Design review of the part built by this model. Coordinates are the model's own, in mm. A direction names the side the tool comes from. Give positions to 0.01 mm unless a question says otherwise; leave off trailing zeros. Loops run counter-clockwise (first coordinate to the right, second up) from the corner with the lowest first, then second, coordinate; pieces in that order, holes last. Notation, with made-up numbers: (81, -25) - (137, -25) arc R38 ccw to (137, 13) - close; hole circle Ø7 at (-6, 89). An arc over 180 degrees is marked (long way). Write each question's results on one line, items separated by ' | '.
Autodesk Inventor part; units mm, degrees
ref_plane "Work Plane1" through (0, 0, 9) normal (0, 0, 1) x (1, 0, 0)
ref_plane "Work Plane2" through (-9, 0, 0) normal (1, 0, 0) x (0, 1, 0)
ref_plane "XZ Plane" through (0, 0, 0) normal (0, 1, 0) x (-1, 0, 0)
sketch "Sketch1" plane through (0, 0, 0) normal (0, 1, 0) x (-1, 0, 0)
  circle A0 centre (0, 0) radius 12.5
  dimension "d0" = 25
extrude "Extrusion1" add sketch "Sketch1" along normal blind 1
chamfer "Chamfer1" distance 0.4 angle 45 1 edges at (12.5, 1, 0)
sketch "Sketch2" plane through (0, 1, 0) normal (0, 1, 0) x (1, 0, 0)
  circle A0 centre (0, 0) radius 12.1
  circle A1 centre (0, 0) radius 9.9
  dimension "d6" = 19.8
extrude "Extrusion2" add sketch "Sketch2" along normal blind 6.5 contours A1
sketch "Sketch3" plane through (0, 7.5, 0) normal (0, 1, 0) x (1, 0, 0)
  circle A0 centre (0, 0) radius 12.5
extrude "Extrusion3" add sketch "Sketch3" along normal blind 1
sketch "Sketch4" plane through (0, 8.5, 0) normal (0, 1, 0) x (1, 0, 0)
  circle A0 centre (0, 0) radius 8.75
  dimension "d14" = 17.5
extrude "Extrusion4" add sketch "Sketch4" along normal blind 9
sketch "Sketch5" plane through (0, 17.5, 0) normal (0, 1, 0) x (1, 0, 0)
  circle A0 centre (0, 0) radius 8.75
  circle A1 centre (0, 0) radius 2.5
  dimension "d17" = 5
extrude "Extrusion5" cut sketch "Sketch5" against normal up to surface (17.5 mm away) contours A1
sketch "Sketch6" plane through (0, 1, 0) normal (0, 1, 0) x (1, 0, 0)
  circle A0 centre (0, 0) radius 9.9
  arc A1 (0.5997, -9.8818) -> (-0.5997, -9.8818) centre (0, -9.9) ccw
  dimension "d20" = 1.2
extrude "Extrusion6" cut sketch "Sketch6" along normal up to surface (6.5 mm away) contours A1 A0 picked at (-0.0236, -9.7001)
pattern_circular "Circular Pattern1" count 32 over 360 about axis through (0, 1, 0) along (0, 1, 0) of "Extrusion6"
ref_plane "Work Plane1" through (0, 0, 9) normal (0, 0, 1) x (1, 0, 0)
ref_plane "Work Plane2" through (-9, 0, 0) normal (1, 0, 0) x (0, 1, 0)
sketch "Sketch7" plane through (-9, 0, 0) normal (1, 0, 0) x (0, 1, 0)
  circle A0 centre (13, 0) radius 1.5
  line L0 (17.5, -8.75) -> (17.5, 8.75)
  point P0 (0, 0)
  dimension "d28" = 3
  dimension "d29" = 4.5
extrude "Extrusion7" cut sketch "Sketch7" along normal blind 7.25
sketch "Sketch8" plane through (0, 0, 9) normal (0, 0, 1) x (1, 0, 0)
  circle A0 centre (0, 13) radius 1.5
  line L0 (12.5, 8.5) -> (-12.5, 8.5)
  point P0 (0, 0)
  dimension "d32" = 3
  dimension "d40" = 4.5
extrude "Extrusion8" cut sketch "Sketch8" against normal blind 8
thread "Thread1"
thread "Thread2"
chamfer "Chamfer3" distance 0.4 angle 45 1 edges at (-12.5, 7.5, 0)
properties part number "PulleyGT2x32x5Bore" material "Aluminum 6061"
Item 1: We need section B-B on z = 0. Give the boundary of the cut face in (x, y).
Output values:
outline: (-12.5, 0) - (-2.5, 0) - (-2.5, 11.5) - (-8.75, 11.5) - (-8.75, 8.5) - (-12.5, 8.5) - (-12.5, 7.9) - (-12.1, 7.5) - (-9.3, 7.5) - (-9.3, 1) - (-12.1, 1) - (-12.5, 0.6) - close; (-8.75, 14.5) - (-2.5, 14.5) - (-2.5, 17.5) - (-8.75, 17.5) - close; (2.5, 0) - (12.5, 0) - (12.5, 0.6) - (12.1, 1) - (9.3, 1) - (9.3, 7.5) - (12.1, 7.5) - (12.5, 7.9) - (12.5, 8.5) - (8.75, 8.5) - (8.75, 17.5) - (2.5, 17.5) - close
Item 2: Wall thickness on probe 1 along Y at (x, z) = (6, -9); probe 2 along Y at (x, z) = (0, 3.5); probe 3 along X at (y, z) = (3.25, -2): over which ranges is each line inside the solid? List them lowest first.
Output values:
probe 1: y = 0 to 1, 7.5 to 8.5 | probe 2: y = 0 to 11.5, 14.5 to 17.5 | probe 3: x = -9.11 to -1.5, 1.5 to 9.11
Item 3: Tool access review of faces 1 (the face through (0, 4.2, -9.3)), 2 (the face through (3.571, 4.204, -8.587)), 3 (the face through (-5.42, 11.5, -0.07)), 4 (the face through (0, 4.2, 9.3)): name each direction out of +Z, -Z, +X, -X, +Y, -Y from which nothing blocks a thin tool from reaching the whole face with its end or side.
Output values:
face 1: -Z | face 2: none | face 3: -X | face 4: +Z
Item 4: We need section C-C on y = 13. Give the boundary of the cut face in (x, z).
Output values:
outline: (-8.62, -1.5) arc R8.75 ccw (long way) to (1.5, 8.62) - (1.5, 2) arc R2.5 cw (long way) to (-2, -1.5) - close; (-8.62, 1.5) - (-2, 1.5) arc R2.5 cw to (-1.5, 2) - (-1.5, 8.62) arc R8.75 ccw to start
Item 5: Draft analysis for pull direction X (two halves, no side actions). For faces 5 (the face through (-11.923, 0.296, -3.755)), 6 (the face through (2, 17.5, 2)), 7 (the face through (-3.547, 4.204, -8.597)), 8 (the face through (-8.597, 4.204, 3.547)), state which applies: +X half, -X half, draft (parallel to the pull), parting line (faces both ways), or undercut.
Output values:
face 5: parting line | face 6: draft | face 7: undercut | face 8: undercut
Item 6: We need section A-A on x = 0. Give the boundary of the cut face in (y, z).
Output values:
outline: (0, -12.5) - (0.6, -12.5) - (1, -12.1) - (1, -9.3) - (7.5, -9.3) - (7.5, -12.1) - (7.9, -12.5) - (8.5, -12.5) - (8.5, -8.75) - (17.5, -8.75) - (17.5, -2.5) - (0, -2.5) - close; (0, 2.5) - (11.5, 2.5) - (11.5, 8.75) - (8.5, 8.75) - (8.5, 12.5) - (7.9, 12.5) - (7.5, 12.1) - (7.5, 9.3) - (1, 9.3) - (1, 12.1) - (0.6, 12.5) - (0, 12.5) - close; (14.5, 2.5) - (17.5, 2.5) - (17.5, 8.75) - (14.5, 8.75) - close
Item 7: Clearance check with flat-ended pins moving along their axes: P1, Ø5, axis at x = -8.5, y = 14, coming from the +Z side; P2, Ø5, axis at x = -2, y = 2, coming from the +Z side; P3, Ø4, axis at y = 12, z = -9.5, coming from the -X side; P4, Ø2.5, axis at x = 0, y = 13, coming from the +Z side. State where each tip first meets the part, or that it passes through.
Output values:
P1: stops at z = 6.37 | P2: stops at z = 12.5 | P3: stops at x = -4.51 | P4: stops at z = -2.17
